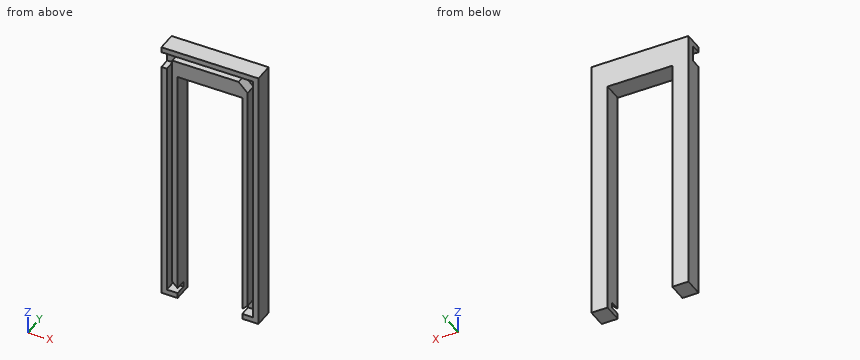
```python
from build123d import *

# Parameters (mm, degrees)
F1_DEPTH = 1.5
F3_DEPTH = 2


with BuildPart() as f1:
    # F0 (on Front) → F1 (new body)
    with BuildSketch(Plane.XZ):
        Polygon((18, 0), (0, 0), (0, -50), (3, -50), (3, -5), (15, -5), (15, -50), (18, -50), align=None)
    extrude(amount=F1_DEPTH)

    # F2 (on face) → F3 (join)
    with BuildSketch(Plane.XZ.offset(1.5)):
        Polygon((0, 0), (0, -1), (17, -1), (17, -49), (15, -49), (15, -50), (18, -50), (18, 0), align=None)
        Polygon((15, -5), (15, -48), (16, -47), (16, -3.693556), (14.306444, -2), (2, -2), (2, -4.21096), (2, -47), (3, -48), (3, -5), align=None)
        Polygon((1, -4), (0, -4), (0, -50), (3, -50), (3, -49), (1, -49), align=None)
    extrude(amount=F3_DEPTH)


solid = f1.part
```
The listing builds one solid part. Answer for the finished solid, in the listing's coordinates (mm). Coordinates: 2 decimals unless noted, no trailing zeros. Loops run counter-clockwise (first coordinate to the right, second up) from the corner with the lowest first, then second, coordinate; pieces in that order, holes last. Notation, with made-up numbers: (72, -5) -> (113, -5) arc R21 ccw to (113, 29) -> close; hole circle Ø11 at (70, -37.5). An arc over 180 degrees is marked (long way). Return JSON: item names as keys, results as strings. Group by question number.
(1) A cutting plane is placed at B-B on x = 6.5. Write down the section's boundary in (y, z), and give its area (3 significant figures).
(2) A cutting plane is placed at D-D on x = 1.5. Write down the section's boundary in (y, z).
(3) A cutting plane is placed at C-C on z = -45.5. Write down the section's boundary in (x, y), and give its area (3 significant figures).
(4) A cutting plane is placed at A-A on y = -2.75. Write down the section's boundary in (x, z), and give its area (3 significant figures).
(5) Given pin 1 Ø1.5 at (x, y) = (14, -1) entering from -Z, flat-ended and moving along its own axis, determine where the tip first touches the part or whether it passes through.
(6) Find the intervals of material crossed by probe 1 along X at (y, z) = (-1.55, -9.5); probe 2 along Z at (x, y) = (11.25, -2.95); probe 3 along X at (y, z) = (-2.9, -4.5), in increasing order. Write a range as from..to.
The answers:
{
 "1": {"outline": "(-3.5, -5) -> (0, -5) -> (0, 0) -> (-3.5, 0) -> (-3.5, -1) -> (-1.5, -1) -> (-1.5, -2) -> (-3.5, -2) -> close", "area": "15.5 mm^2"},
 "2": {"outline": "(-3.5, -50) -> (0, -50) -> (0, 0) -> (-3.5, 0) -> (-3.5, -1) -> (-1.5, -1) -> (-1.5, -49) -> (-3.5, -49) -> close"},
 "3": {"outline": "(0, -3.5) -> (1, -3.5) -> (1, -1.5) -> (2, -1.5) -> (2, -3.5) -> (3, -3.5) -> (3, 0) -> (0, 0) -> close; (15, -3.5) -> (16, -3.5) -> (16, -1.5) -> (17, -1.5) -> (17, -3.5) -> (18, -3.5) -> (18, 0) -> (15, 0) -> close", "area": "17.0 mm^2"},
 "4": {"outline": "(0, -50) -> (3, -50) -> (3, -49) -> (1, -49) -> (1, -4) -> (0, -4) -> close; (0, -1) -> (17, -1) -> (17, -49) -> (15, -49) -> (15, -50) -> (18, -50) -> (18, 0) -> (0, 0) -> close; (2, -47) -> (3, -48) -> (3, -5) -> (15, -5) -> (15, -48) -> (16, -47) -> (16, -3.69) -> (14.31, -2) -> (2, -2) -> close", "area": "243 mm^2"},
 "5": {"pin 1": "stops at z = -5"},
 "6": {"probe 1": "x = 0..1, 2..3, 15..16, 17..18", "probe 2": "z = -5..-2, -1..0", "probe 3": "x = 0..1, 2..16, 17..18"}
}
